from build123d import *

# Parameters (mm, degrees)
F0_R     = 9.1313
F1_DEPTH = 55.1688
F2_R     = 4.590873
F3_DEPTH = 152.4


with BuildPart() as f1:
    # F0 (on Front) → F1 (new body)
    with BuildSketch(Plane.XZ):
        with BuildLine():
            ThreePointArc((5.690516, 60.901123), (8.49944, 57.841701), (12.495555, 56.709803))
            Line((12.495555, 56.709803), (57.916488, 56.709803))
            ThreePointArc((57.916488, 56.709803), (59.71254, 57.453752), (60.456488, 59.249803))
            Line((60.456488, 59.249803), (60.456488, 62.247003))
            ThreePointArc((60.456488, 62.247003), (59.71254, 64.043054), (57.916488, 64.787003))
            Line((57.916488, 64.787003), (41.860021, 64.787003))
            ThreePointArc((41.860021, 64.787003), (36.75553, 67.359878), (35.787486, 72.993563))
            Line((35.787486, 72.993563), (76.573475, 206.398524))
            Line((76.573475, 206.398524), (82.764438, 256.819868))
            Line((82.764438, 256.819868), (82.764438, 327.140741))
            ThreePointArc((82.764438, 327.140741), (79.649249, 335.472691), (71.831936, 339.717145))
            Line((71.831936, 339.717145), (39.319936, 344.286409))
            Line((39.319936, 344.286409), (4.80626, 296.78241))
            ThreePointArc((4.80626, 296.78241), (-3.021214, 291.785261), (-12.157108, 293.451485))
            Line((-12.157108, 293.451485), (-24.39685, 301.034975))
            ThreePointArc((-24.39685, 301.034975), (-26.76481, 302.181534), (-29.318204, 302.815581))
            Line((-29.318204, 302.815581), (-50.053234, 305.729699))
            Line((-50.053234, 305.729699), (-51.601562, 294.712769))
            Line((-51.601562, 294.712769), (-31.353263, 291.867056))
            ThreePointArc((-31.353263, 291.867056), (-26.860403, 290.340444), (-23.241498, 287.271263))
            ThreePointArc((-23.241498, 287.271263), (-18.05967, 277.295323), (-17.18101, 266.08824))
            Line((-17.18101, 266.08824), (-22.943347, 219.157768))
            Line((-22.943347, 219.157768), (-13.954531, 100.743315))
            ThreePointArc((-13.954531, 100.743315), (-13.783375, 99.766758), (-13.425797, 98.842044))
            Line((-13.425797, 98.842044), (5.690516, 60.901123))
        make_face()
        with BuildLine():
            ThreePointArc((0, 107.610365), (-3.195116, 104.203), (-6.80066, 107.172673))
            Line((-6.80066, 107.172673), (-13.422605, 194.407079))
            ThreePointArc((-13.422605, 194.407079), (-12.050117, 198.853564), (-8.01427, 201.170218))
            Line((-8.01427, 201.170218), (-7.273448, 201.27911))
            ThreePointArc((-7.273448, 201.27911), (-2.199181, 199.802153), (0, 194.996615))
            Line((0, 194.996615), (0, 107.610365))
        make_face(mode=Mode.SUBTRACT)
        with Locations((16.958988, 74.324703)):
            Circle(F0_R, mode=Mode.SUBTRACT)
        with BuildLine():
            Line((21.773085, 205.443941), (22.146465, 205.498823))
            Line((22.146465, 205.498823), (50.683851, 201.488155))
            ThreePointArc((50.683851, 201.488155), (59.627424, 195.735456), (61.061423, 185.19863))
            Line((61.061423, 185.19863), (31.771058, 89.394163))
            ThreePointArc((31.771058, 89.394163), (29.797055, 87.330417), (26.963626, 87.687371))
            ThreePointArc((26.963626, 87.687371), (20.942359, 90.395582), (14.363594, 90.952282))
            ThreePointArc((14.363594, 90.952282), (11.946985, 91.777794), (10.919982, 94.115899))
            Line((10.919982, 94.115899), (10.919982, 192.878951))
            ThreePointArc((10.919982, 192.878951), (14.008905, 201.18059), (21.773085, 205.443941))
        make_face(mode=Mode.SUBTRACT)
        with BuildLine():
            Line((55.24467, 210.414482), (23.465019, 214.880821))
            ThreePointArc((23.465019, 214.880821), (21.657413, 215.004353), (19.850623, 214.869406))
            Line((19.850623, 214.869406), (1.98934, 212.244021))
            ThreePointArc((1.98934, 212.244021), (-8.730453, 215.722663), (-12.462892, 226.356751))
            Line((-12.462892, 226.356751), (-8.740444, 256.673662))
            ThreePointArc((-8.740444, 256.673662), (0.247859, 267.299954), (13.580182, 263.305356))
            Line((13.580182, 263.305356), (18.524945, 257.432113))
            ThreePointArc((18.524945, 257.432113), (22.092313, 254.498804), (26.472736, 253.035143))
            Line((26.472736, 253.035143), (60.340027, 248.275405))
            ThreePointArc((60.340027, 248.275405), (68.648116, 243.430271), (71.177865, 234.15126))
            Line((71.177865, 234.15126), (69.617505, 221.443146))
            ThreePointArc((69.617505, 221.443146), (64.743439, 212.915299), (55.24467, 210.414482))
        make_face(mode=Mode.SUBTRACT)
        with BuildLine():
            Line((59.405725, 255.152563), (31.327721, 259.098669))
            ThreePointArc((31.327721, 259.098669), (26.947298, 260.562331), (23.37993, 263.495639))
            Line((23.37993, 263.495639), (11.885566, 277.148304))
            ThreePointArc((11.885566, 277.148304), (8.908962, 284.87405), (11.32634, 292.792611))
            Line((11.32634, 292.792611), (34.283751, 324.390777))
            ThreePointArc((34.283751, 324.390777), (36.939866, 326.503546), (40.304758, 326.946542))
            Line((40.304758, 326.946542), (68.204987, 323.025421))
            ThreePointArc((68.204987, 323.025421), (72.113644, 320.903194), (73.671238, 316.737219))
            Line((73.671238, 316.737219), (73.671238, 266.044077))
            ThreePointArc((73.671238, 266.044077), (68.814325, 257.61746), (59.405725, 255.152563))
        make_face(mode=Mode.SUBTRACT)
    extrude(amount=F1_DEPTH)

    # F2 (on face) → F3 (cut)
    with BuildSketch(Plane(origin=(48.210692, 0, 343.036895), x_dir=(0.990268, 0, -0.139173), z_dir=(0.139173, 0, 0.990268))):
        with Locations((0, -27.5844)):
            Circle(F2_R)
    extrude(amount=-F3_DEPTH, mode=Mode.SUBTRACT)


solid = f1.part
Input: part model. Units: mm. Frame: model coordinates. A direction names the side the tool comes from. Coordinates: 2 decimals unless noted, no trailing zeros. Loops run counter-clockwise (first coordinate to the right, second up) from the corner with the lowest first, then second, coordinate; pieces in that order, holes last.
Q1. Cut plane B-B (z = 156). Output: boundary loops of the cut face in (x, y).
Q2. Contact query for flat-ended pins moving along their axis: pin 1 (2 mm diameter, centred on x = 43, y = -26.5, fed in from +Z); pin 2 (8 mm diameter, centred on x = -19, y = -21, fed in from +Z); pin 3 (6 mm diameter, centred on x = -2.5, y = -15.5, fed in from +Z). Output: stop coordinate, or through.
Q3. Cut plane C-C (y = -41). Give the number of separate pieces and of enclosed holes in the cut face, then the cut area to 3 significant figures.
Q4. Cut plane D-D (x = -40.5). Output: boundary loops of the cut face in (y, z).
Q5. Set-up query: faces 1 (the face through (-20.022, -27.198, 242.952)), 2 (the face through (22.305, -27.198, 320.867)), 3 (the face through (-10.63, -27.2, 241.3)), 4 (the face through (79.626, -27.198, 231.256)). Return all of +Z, -Z, +X, -X, +Y, -Y with unobstructed straight access to the full face (end or side cutting, diameter ignored); none if empty.
Q6. Draft query along Z for faces 5 (the face through (20, -55.169, 212)), 6 (the face through (64.85, -27.2, 213)), 7 (the face through (-26.919, -27.198, 290.373)). Return one class per face: +Z half, -Z half, draft (parallel to the pull), parting line (faces both ways), or undercut.
Q7. Cut plane A-A (z = 273). Output: boundary loops of the cut face in (x, y), then the cut area to 3 significant figures.
Q8. Material intervals for line 1 (X direction, y = -3.5, z = 108); line 2 (Z direction, x = 21, y = -24.5); line 3 (Z direction, x = -1.5, y = -35.5), sorted ascending.
Working result:
1. outline: (-18.15, -55.17) - (-10.51, -55.17) - (-10.51, 0) - (-18.15, 0) - close; (0, -55.17) - (10.92, -55.17) - (10.92, 0) - (0, 0) - close; (52.13, -55.17) - (61.17, -55.17) - (61.17, 0) - (52.13, 0) - close
2. pin 1: stops at z = 343.91
2. pin 2: stops at z = 300.17
2. pin 3: stops at z = 293.04
3. separate pieces: 1
3. enclosed holes: 5
3. area: 9,870 mm2
4. outline: (-55.17, 293.15) - (0, 293.15) - (0, 304.39) - (-55.17, 304.39) - close
5. face 1: -X, +Y, -Y
5. face 2: +Z, +Y, -Y
5. face 3: +Y, -Y
5. face 4: -Z, +X, +Y, -Y
6. face 5: draft
6. face 6: undercut
6. face 7: -Z half
7. outline: (-17.18, -55.17) - (15.38, -55.17) - (15.38, 0) - (-17.18, 0) - close; (73.67, -55.17) - (82.76, -55.17) - (82.76, 0) - (73.67, 0) - close
7. area: 2,300 mm2
8. line 1: x = -14.51 to -6.86, 0 to 10.92, 37.46 to 46.49
8. line 2: z = 56.71 to 66.14, 82.51 to 90.38, 205.31 to 214.99, 255.18 to 266.32, 306.11 to 319.07
8. line 3: z = 75.17 to 104.78, 199.1 to 212.22, 266.64 to 292.18
